Build history of the part. All positions in model axes, mm. Give positions to 0.01 mm unless a question says otherwise; leave off trailing zeros. Order: outer loops, then holes, each group sorted by start corner. A loop starts at its lowest first (then second) coordinate and runs counter-clockwise, first axis right, second up. Notation, with made-up numbers: M 6,80.25 L 56,80.25 A23 ccw 56,118.25 Z; hole C 17,54.25 d2. An arc over 180 degrees is marked long. Answer as CSV lines item,"result".
from build123d import *

# Parameters (mm, degrees)
SKETCH1_W           = 218
SKETCH1_H           = 12.3
SKETCH1_R           = 1.25
BOSS_EXTRUDE1_DEPTH = 6.25
SKETCH2_R           = 1.25
CUT_EXTRUDE1_DEPTH  = 8
FILLET1_R           = 1


with BuildPart() as part:
    # Sketch1 → Boss-Extrude1 (new body)
    with BuildSketch(Plane.XY):
        with Locations((109, 6.15)):
            Rectangle(SKETCH1_W, SKETCH1_H)
        with Locations((143, 6.15)):
            Circle(SKETCH1_R, mode=Mode.SUBTRACT)
        with Locations((99, 6.15)):
            Circle(SKETCH1_R, mode=Mode.SUBTRACT)
    extrude(amount=BOSS_EXTRUDE1_DEPTH)

    # Sketch2 → Cut-Extrude1 (cut)
    with BuildSketch(Plane(origin=(0, 12.3, 0), x_dir=(1, 0, 0), z_dir=(0, 1, 0))):
        with Locations(Location((214.5, -3.125, 0), (0, 0, 270))):
            Circle(SKETCH2_R)
        with Locations(Location((177, -3.125, 0), (0, 0, 270))):
            Circle(SKETCH2_R)
        with Locations(Location((3.5, -3.125, 0), (0, 0, 90))):
            Circle(SKETCH2_R)
        with Locations(Location((41, -3.125, 0), (0, 0, 90))):
            Circle(SKETCH2_R)
    extrude(amount=-CUT_EXTRUDE1_DEPTH, mode=Mode.SUBTRACT)

    # Fillet1
    fillet1_edges = [part.edges().sort_by_distance(p)[0] for p in [
        (109, 12.3, 6.25),
        (109, 12.3, 0),
        (109, 0, 0),
        (109, 0, 6.25),
    ]]
    fillet(fillet1_edges, radius=FILLET1_R)


with BuildPart() as part_1:
    # Body-Move/Copy1: moved
    add(part.part.moved(Location((0, 5e-08, 6.25))))


solid = part_1.part
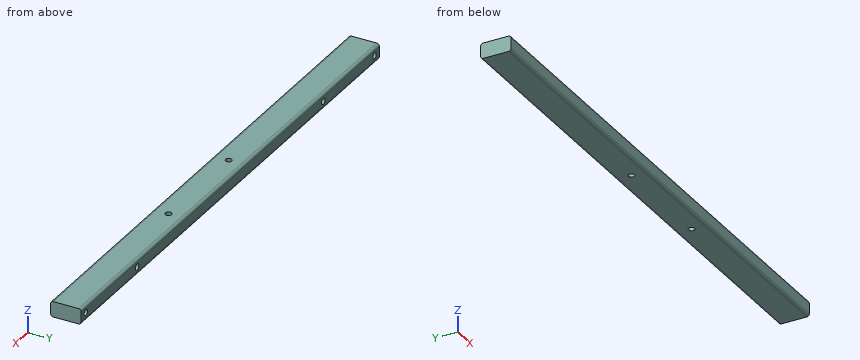
Item 1: Band-saw the part on A-A (z = 9.5). Give the cut face in (x, y).
Geometry says:
outline,"M 0,0 L 218,0 L 218,12.3 L 215.74,12.3 L 215.74,4.3 L 213.26,4.3 L 213.26,12.3 L 178.24,12.3 L 178.24,4.3 L 175.76,4.3 L 175.76,12.3 L 42.24,12.3 L 42.24,4.3 L 39.76,4.3 L 39.76,12.3 L 4.74,12.3 L 4.74,4.3 L 2.26,4.3 L 2.26,12.3 L 0,12.3 Z; hole C 99,6.15 d2.5; hole C 143,6.15 d2.5"
Item 2: Drop flat-ended pins along their axis: pin 1 (1.2 mm diameter, centred on x = 3, z = 9.5, fed in from +Y); pin 2 (2 mm diameter, centred on x = 143, y = 6.15, fed in from -Z). Give the stop position or say it passes through.
Geometry says:
pin 1,"stops at y = 4.3"
pin 2,"passes through"
Item 3: Probe line 1 along X through (y, z) = (10, 8.25); line 2 along X through (y, z) = (6.5, 11.5); line 3 along Y through (x, z) = (143, 8.5). List the from-to ranges inside material, lowest first. Write a range as from..to.
Geometry says:
line 1,"x = 0..2.96, 4.04..40.46, 41.54..176.46, 177.54..213.96, 215.04..218"
line 2,"x = 0..97.8, 100.2..141.8, 144.2..218"
line 3,"y = 0..4.9, 7.4..12.3"
